Could you check a few things on this drawing? It's one solid part, dimensions in mm from its lowest x, y, z. A direction names the side the tool comes from. Coordinates: 2 decimals unless noted, no trailing zeros. Write each loop counter-clockwise with the first axis right and the second up, starting at its lowest first coordinate (ties: lowest second). Pieces come first, ordered by that corner, then holes. Notation, with made-up numbers: (29, 52.25) - (55, 52.25) arc R7 cw to (55, 58.25) - close; hole circle Ø11 at (33, 9). An arc over 180 degrees is marked (long way). Use one line per item in the form item = value. Start each with the question number.
(1) If we section it at B-B on x = 6.75: Please give me the cut outline in (y, z) (1 decimal).
(2) If we section it at A-A on y = 2: Please give me the cut outline in (x, z) (1 decimal).
(3) If I drill on probe 1 along Z at (x, y) = (4.25, 2.5); probe 2 along Y at (x, z) = (7, 8) (1 decimal); probe 3 along X at (y, z) = (13.5, 4.25), over which ranges is the centre line in solid material (lowest first)? Write a range as from..to.
(4) On a 3-axis mill with a long thin cutter (end or side, diameter ignored), from which of +Z, -Z, +X, -X, +Y, -Y can I reach the whole of each face in a straight line? I mean the marked faces 1, 2, 3, 4 and 5. Say none if no direction works.
(5) If we section it at C-C on z = 3.75: Please give me the cut outline in (x, y) (1 decimal), then the cut area to 3 significant figures.
(6) If we section it at D-D on y = 13.5: Please give me the cut outline in (x, z).
(7) Thinking about a two-plate mould opening in X: for the marked faces 6, 7 and 8, which applies, pulls with the +X half, pulls with the -X half, needs draft (parallel to the pull), parting line crosses it, or undercut?
(8) For pin 1 Ø1 at (x, z) = (7, 3.5) entering from -Y (1 decimal); pin 2 Ø2 at (y, z) = (14.5, 3) entering from -X; pin 3 Ø1.2 at (x, y) = (4.5, 15.5) entering from -Z, each with a flat end and sliding along its axis, tell me the tip position at first contact or that it passes through.
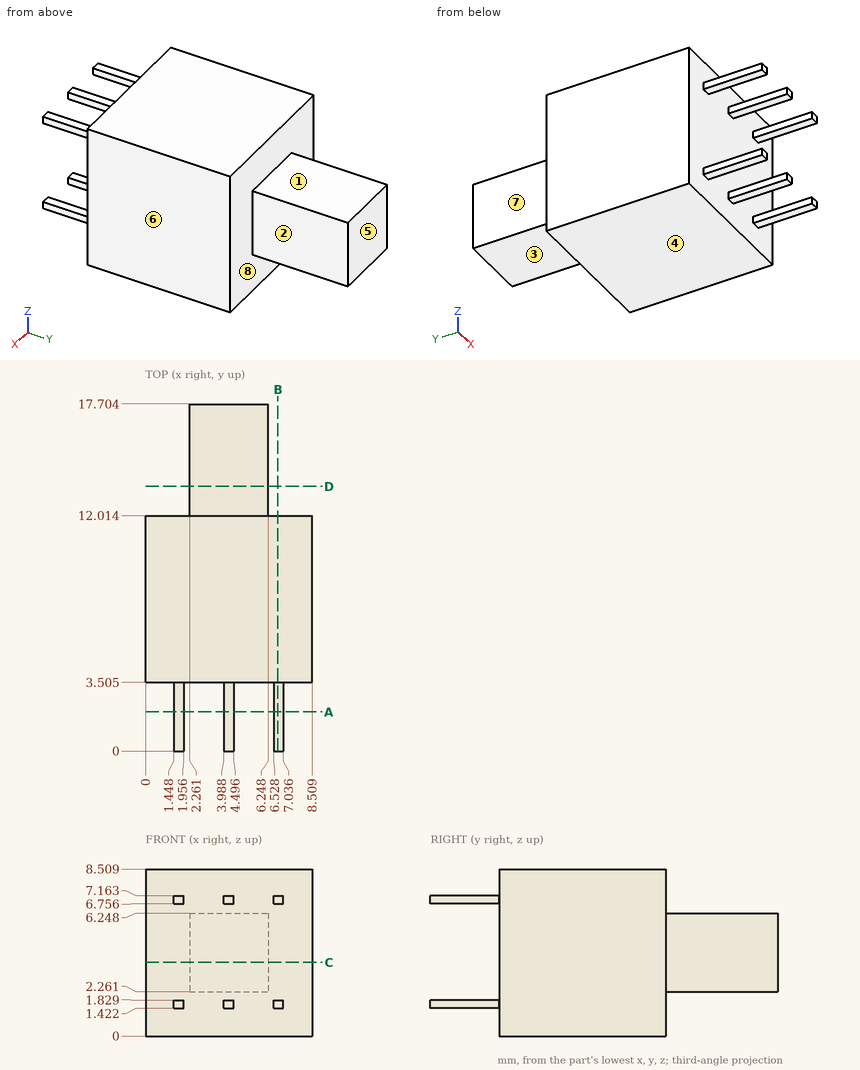
Reported:
q1.outline = (0, 1.4) - (3.5, 1.4) - (3.5, 0) - (12, 0) - (12, 8.5) - (3.5, 8.5) - (3.5, 7.2) - (0, 7.2) - (0, 6.8) - (3.5, 6.8) - (3.5, 1.8) - (0, 1.8) - close
q2.outline = (1.4, 1.4) - (2, 1.4) - (2, 1.8) - (1.4, 1.8) - close; (1.4, 6.8) - (2, 6.8) - (2, 7.2) - (1.4, 7.2) - close; (4, 1.4) - (4.5, 1.4) - (4.5, 1.8) - (4, 1.8) - close; (4, 6.8) - (4.5, 6.8) - (4.5, 7.2) - (4, 7.2) - close; (6.5, 1.4) - (7, 1.4) - (7, 1.8) - (6.5, 1.8) - close; (6.5, 6.8) - (7, 6.8) - (7, 7.2) - (6.5, 7.2) - close
q3.probe_1 = 1.42..1.83, 6.76..7.16
q3.probe_2 = 3.5..12
q3.probe_3 = 2.26..6.25
q4.face_1 = +Z, +X, -X, +Y
q4.face_2 = +Z, -Z, +X, +Y
q4.face_3 = -Z, +X, -X, +Y
q4.face_4 = -Z, +X, -X, +Y, -Y
q4.face_5 = +Z, -Z, +X, -X, +Y
q5.outline = (0, 3.5) - (8.5, 3.5) - (8.5, 12) - (6.2, 12) - (6.2, 17.7) - (2.3, 17.7) - (2.3, 12) - (0, 12) - close
q5.area = 95.1 mm2
q6.outline = (2.26, 2.26) - (6.25, 2.26) - (6.25, 6.25) - (2.26, 6.25) - close
q7.face_6 = pulls with the +X half
q7.face_7 = pulls with the -X half
q7.face_8 = needs draft
q8.pin_1 = 3.5
q8.pin_2 = 2.26
q8.pin_3 = 2.26
